Geometry: final body of the model. Coordinates: model frame, mm. Give positions to 0.01 mm unless a question says otherwise; leave off trailing zeros. Write each loop counter-clockwise with the first axis right and the second up, starting at its lowest first coordinate (ties: lowest second). Pieces come first, ordered by that corner, then holes. Notation, with made-up numbers: M 23.25,-26.5 L 67.25,-26.5 A21 ccw 67.25,-2.5 Z; hole C 62.5,67 d10. An arc over 180 degrees is marked long. Use a Markdown table: item, result. Add a question column.
(1) Draft query along X for faces 1 (the cylindrical face through (-0.434, -1.521, 38.548)), 2 (the flat face through (0, 0, 1)), 3 (the flat face through (23, -1, -1)). Return one class per face: released by +X, released by -X, zero draft, split by the parting line, or undercut.
(2) Cut plane D-D (z = -13.5). Output: boundary loops of the cut face in (x, y).
(3) Cut plane B-B (y = -0.75). Output: boundary loops of the cut face in (x, z), plus the area to 3 significant figures.
(4) Cut plane A-A (z = 40.5). Output: boundary loops of the cut face in (x, y).
(5) Pin query (flat end, axial travel): pin 1 Ø0.8 at (y, z) = (-3.5, 6.5) entering from -X; pin 2 Ø6.5 at (x, z) = (0, 30) entering from -Y; pin 3 Ø0.8 at (y, z) = (-3.5, 17.5) entering from +X. Return the tip coordinate at first contact, or that it passes through.
(6) Cut plane C-C (x = 8.5). Output: boundary loops of the cut face in (y, z), plus the area to 3 significant figures.
(7) Material intervals for L1, parallel to Z at x = 0, y = -2; L2, parallel to Y at x = -20, z = 32; L3, parallel to X at y = -3.2, z = -15, sorted ascending.
```python
from build123d import *

# Parameters (mm, degrees)
F0_W     = 46
F0_H     = 86
F1_DEPTH = 3
F2_W     = 39
F2_H     = 73
F3_DEPTH = 1
F4_R     = 2
F5_DEPTH = 3
F6_R     = 3.5
F7_DEPTH = 4


with BuildPart() as f1:
    # F0 (on Front) → F1 (new body)
    with BuildSketch(Plane.XZ):
        Rectangle(F0_W, F0_H)
    extrude(amount=F1_DEPTH)

    # F2 (on face) → F3 (join)
    with BuildSketch(Plane.XZ.offset(3)):
        Rectangle(F2_W, F2_H)
    extrude(amount=F3_DEPTH)

    # F4 (on face) → F5 (cut)
    with BuildSketch(Plane.XZ.offset(3)):
        with Locations((0, 40.5)):
            Circle(F4_R)
        with Locations((0, -40.5)):
            Circle(F4_R)
    extrude(amount=-F5_DEPTH, mode=Mode.SUBTRACT)

    # F6 (on face) → F7 (cut)
    with BuildSketch(Plane.XZ.offset(4)):
        with Locations((0, 30)):
            Circle(F6_R)
    extrude(amount=-F7_DEPTH, mode=Mode.SUBTRACT)


solid = f1.part
```
Answer list:
| question | item | result |
|---|---|---|
| 1 | face 1 | undercut |
| 1 | face 2 | zero draft |
| 1 | face 3 | released by +X |
| 2 | outline | M -23,-3 L -19.5,-3 L -19.5,-4 L 19.5,-4 L 19.5,-3 L 23,-3 L 23,0 L -23,0 Z |
| 3 | outline | M -23,-43 L 23,-43 L 23,43 L -23,43 Z; hole C 0,30 d7; hole C 0,-40.5 d4; hole C 0,40.5 d4 |
| 3 | area | 3,890 mm² |
| 4 | outline | M -23,-3 L -2,-3 L -2,0 L -23,0 Z; M 2,-3 L 23,-3 L 23,0 L 2,0 Z |
| 5 | pin 1 | x = -19.5 |
| 5 | pin 2 | through |
| 5 | pin 3 | x = 19.5 |
| 6 | outline | M -4,-36.5 L -3,-36.5 L -3,-43 L 0,-43 L 0,43 L -3,43 L -3,36.5 L -4,36.5 Z |
| 6 | area | 331 mm² |
| 7 | L1 | -43 to -42.5, -38.5 to 26.5, 33.5 to 38.5, 42.5 to 43 |
| 7 | L2 | -3 to 0 |
| 7 | L3 | -19.5 to 19.5 |
